from build123d import *


with BuildPart() as f1:
    # F0 (on Front) → F1 (revolve)
    with BuildSketch(Plane.XZ):
        with BuildLine():
            Line((0, 25.350947), (0, 0))
            Line((0, 0), (0, -4.13963))
            Line((0, -4.13963), (54.233268, -4.13963))
            Line((54.233268, -4.13963), (54.233268, 15.87638))
            ThreePointArc((54.233268, 15.87638), (53.160671, 18.526423), (50.546798, 19.684377))
            Line((50.546798, 19.684377), (46.35951, 19.820212))
            ThreePointArc((46.35951, 19.820212), (44.138408, 20.625078), (42.818762, 22.584578))
            ThreePointArc((42.818762, 22.584578), (41.450118, 24.581698), (39.154484, 25.350947))
            Line((39.154484, 25.350947), (0, 25.350947))
        make_face()
    revolve(axis=Axis((0, 0, 12.675473), (0, 0, 1)))


solid = f1.part
The model under review builds one solid part; all positions refer to its coordinate system, in mm. A direction names the side the tool comes from. Round coordinates to 2 decimals unless told otherwise and drop trailing zeros. Loops run counter-clockwise (first coordinate to the right, second up) from the corner with the lowest first, then second, coordinate; pieces in that order, holes last. Notation, with made-up numbers: (1.25, -38.5) -> (56.25, -38.5) arc R21 cw to (56.25, -17.5) -> close; hole circle Ø9 at (66, -6). An arc over 180 degrees is marked (long way). Answer as CSV lines item,"result".
1) For P1, Ø4, axis at x = -2, z = 21, coming from the +Y side; P2, Ø6, axis at y = -7, z = 13, coming from the -X side; P3, Ø2, axis at y = 21.5, z = 9.5, coming from the -X side, all flat-tipped, find the tip position at first contact; note any pin that passes through.
Geometry results:
P1,"stops at y = 52.57"
P2,"stops at x = -54.09"
P3,"stops at x = -50.21"
2) To check wall thickness, follow line 1 along Z through (x, y) = (-30, -40); line 2 along Z through (x, y) = (13.5, 45); line 3 along Y through (x, z) = (34, 22.75). State the ranges of each line that lie inside material, in increasing order. Write a range as from..to.
Geometry results:
line 1,"z = -4.14..19.7"
line 2,"z = -4.14..19.8"
line 3,"y = -25.94..25.94"
3) Add section D-D on z = 18. Write out the cut boundary in (x, y).
Geometry results:
outline,"circle Ø107.17 at (0, 0)"
4) Add section A-A on x = 0. Write out the cut boundary in (y, z), plus the area to 3 significant figures.
Geometry results:
outline,"(-54.23, -4.14) -> (54.23, -4.14) -> (54.23, 15.88) arc R3.81 ccw to (50.55, 19.68) -> (46.36, 19.82) arc R3.81 cw to (42.82, 22.58) arc R3.81 ccw to (39.15, 25.35) -> (-39.15, 25.35) arc R3.81 ccw to (-42.82, 22.58) arc R3.81 cw to (-46.36, 19.82) -> (-50.55, 19.68) arc R3.81 ccw to (-54.23, 15.88) -> close"
area,"3,060 mm²"
5) Add section C-C on z = 12.5. Write out the cut boundary in (x, y).
Geometry results:
outline,"circle Ø108.47 at (0, 0)"
6) Tool access review of faces 1 (the face through (44.413, 13.986, 19.814)), 2 (the face through (-1, 1, 25.351)): name each direction out of +Z, -Z, +X, -X, +Y, -Y from which nothing blocks a thin tool from reaching the whole face with its end or side.
Geometry results:
face 1,"+Z"
face 2,"+Z, +X, -X, +Y, -Y"
